Verification items for the finished model (mm, model axes). Coordinates: 2 decimals unless noted, no trailing zeros. Use CSV: the item, a comma, the result in double quotes. Start each with the question number.
Autodesk Inventor part; units mm, degrees
ref_plane "YZ Plane" through (0, 0, 0) normal (1, 0, 0) x (0, 1, 0)
ref_plane "XZ Plane" through (0, 0, 0) normal (0, 1, 0) x (-1, 0, 0)
ref_plane "XY Plane" through (0, 0, 0) normal (0, 0, 1) x (1, 0, 0)
sketch "Szkic1" plane through (0, 0, 0) normal (1, 0, 0) x (0, 1, 0)
  line L0 (0, 0) -> (15, 0) construction
  line L1 (15, 0) -> (50, 0) construction
  line L2 (50, 0) -> (65, 0) construction
  line L3 (0, 0) -> (-50, 0) construction
  line L4 (-50, 0) -> (-60, 0) construction
  line L5 (-60, 10) -> (-60, -10) construction
  circle A0 centre (50, 0) radius 1.5
  circle A1 centre (15, 0) radius 1.5
  circle A2 centre (-60, -10) radius 1.5
  circle A3 centre (-60, 10) radius 1.5
  line L6 (-60, 0) -> (-64.5, 0) construction
  line L7 (-64.5, 0) -> (-70, 0) construction
  line L8 (-70, 0) -> (-95, 0) construction
  line L9 (-64.5, 7.5) -> (-64.5, -7.5)
  line L10 (-64.5, -7.5) -> (-70, -7.5)
  line L11 (-70, -7.5) -> (-70, 7.5)
  line L12 (-70, 7.5) -> (-64.5, 7.5)
  circle A4 centre (-95, 0) radius 2.5 construction
  line L13 (-95, 0) -> (-89, 0) construction
  line L14 (-89, 0) -> (-86.5, 0) construction
  line L15 (-86.5, 0) -> (-84, 0) construction
  circle A5 centre (-86.5, 0) radius 1.25
  line L16 (-95, 0) -> (-113, 0) construction
  line L17 (-113, 0) -> (-115.5, 0) construction
  line L18 (-115.5, 0) -> (-118, 0) construction
  circle A6 centre (-115.5, 0) radius 1.25
  line L19 (-89, 0) -> (-88.7, 0) construction
  line L20 (-113, 0) -> (-113.3, 0) construction
  line L21 (-113.3, 6.5) -> (-113.3, -6.5)
  line L22 (-113.3, -6.5) -> (-88.7, -6.5)
  line L23 (-88.7, -6.5) -> (-88.7, 6.5)
  line L24 (-88.7, 6.5) -> (-113.3, 6.5)
  line L25 (-84, 0) -> (-83.7, 0) construction
  line L26 (-83.7, 6.5) -> (-83.7, -6.5)
  line L27 (-83.7, -6.5) -> (-88.7, -6.5)
  line L28 (-83.7, 6.5) -> (-88.7, 6.5)
  line L29 (-118, 0) -> (-118.3, 0) construction
  line L30 (-118.3, 6.5) -> (-118.3, -6.5)
  line L31 (-118.3, -6.5) -> (-113.3, -6.5)
  line L32 (-113.3, 6.5) -> (-118.3, 6.5)
  line L33 (-118.3, 0) -> (-198.3, 0) construction
  line L34 (15, 15) -> (15, -15) construction
  line L35 (50, 0) -> (37, 0) construction
  line L36 (37, 2.5) -> (37, -2.5)
  line L37 (37, -2.5) -> (34, -2.5)
  line L38 (34, -2.5) -> (34, 2.5)
  line L39 (34, 2.5) -> (37, 2.5)
  line L40 (34, 0) -> (31, 0) construction
  line L41 (31, 2.5) -> (31, -2.5)
  line L42 (31, -2.5) -> (28, -2.5)
  line L43 (28, -2.5) -> (28, 2.5)
  line L44 (28, 2.5) -> (31, 2.5)
  line L45 (-198.3, 15) -> (-198.3, -15)
  line L46 (-198.3, -15) -> (15, -15)
  line L47 (15, 15) -> (-198.3, 15)
  ellipse E0 centre (15, 0) end of major axis (15, 15) minor radius 50 (15, -15) -> (15, 15) ccw
  dimension "d0" = 15
  dimension "d1" = 35
  dimension "d2" = 15
  dimension "d3" = 50
  dimension "d4" = 10
  dimension "d5" = 20
  dimension "d6" = 3
  dimension "d7" = 3
  dimension "d8" = 3
  dimension "d9" = 3
  dimension "d10" = 4.5
  dimension "d11" = 5.5
  dimension "d12" = 25
  dimension "d13" = 15
  dimension "d14" = 5.5
  dimension "d15" = 5
  dimension "d16" = 6
  dimension "d17" = 2.5
  dimension "d18" = 2.5
  dimension "d19" = 2.5
  dimension "d20" = 18
  dimension "d21" = 2.5
  dimension "d22" = 2.5
  dimension "d23" = 2.5
  dimension "d24" = 0.3
  dimension "d25" = 0.3
  dimension "d26" = 13
  dimension "d27" = 24.6
  dimension "d28" = 0.3
  dimension "d29" = 0.3
  dimension "d30" = 80
  dimension "d31" = 30
  dimension "d32" = 13
  dimension "d33" = 5
  dimension "d34" = 3
  dimension "d35" = 3
  dimension "d36" = 5
  dimension "d37" = 3
  dimension "d38" = 30
  dimension "d39" = 213.3
extrude "Wyciągnięcie proste1" add sketch "Szkic1" along normal blind 10 contours L47 E0 L46 L45
extrude "Wyciągnięcie proste2" add sketch "Szkic1" along normal blind 4 contours L21 L31 L30 L32 | L28 L26 L27 L23
properties part number "008-002"
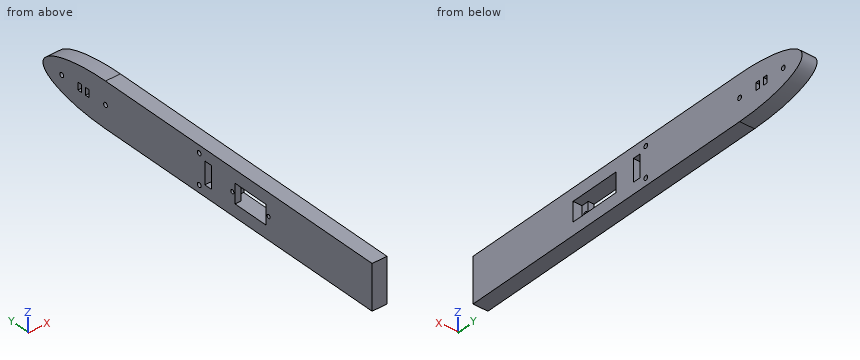
Q1. Scan lines: line 1 along Z through (x, y) = (5, -90.5); line 2 along Z through (x, y) = (1.05, -86.5); line 3 along Y through (x, z) = (2, -6.75). Record each from-to range of solid material in increasing order. Write a range as from..to.
Q2. Gauge pin test, flat ends, axial feed: pin 1 (2 mm diameter, centred on y = -86.5, z = 0, fed in from +X); pin 2 (0.9 mm diameter, centred on x = 7, y = 29, fed in from +Z); pin 3 (3 mm diameter, centred on y = -115.5, z = 0, fed in from +X); pin 4 (3.5 mm diameter, centred on x = 7, y = 30, fed in from -Z). Record the tip position at first contact, or that the pin passes through.
Q3. Cross-section at A-A (x = 7.25). State how many separate pieces and enclosed holes the cut face has, plus the area to 3 significant figures.
Reply:
1,line 1,"-15..-6.5, 6.5..15"
1,line 2,"-15..-1.25, 1.25..15"
1,line 3,"-198.3..-70, -64.5..59.65"
2,pin 1,"through"
2,pin 2,"z = 14.44"
2,pin 3,"x = 4"
2,pin 4,"z = -14.46"
3,separate pieces,"1"
3,enclosed holes,"8"
3,area,"6,990 mm^2"
